Geometry check sheet. Reference: the model listing, model coordinates, mm. A direction names the side the tool comes from. Round coordinates to 2 decimals unless told otherwise and drop trailing zeros. Write each loop counter-clockwise with the first axis right and the second up, starting at its lowest first coordinate (ties: lowest second). Pieces come first, ordered by that corner, then holes. Notation, with made-up numbers: M -24,-39.75 L 9,-39.75 A21 cw 9,-3.75 Z; hole C -5,0.5 d9. An arc over 180 degrees is marked long. One line per item, written item: value. Start each with the question number.
1. Section check D-D (y = -8.5). Record the boundary of the cut face in (x, z).
2. Scan lines: probe 1 along Z at (x, y) = (68.5, -9.25); probe 2 along Z at (x, y) = (0, -7); probe 3 along Z at (x, y) = (46.5, -4). Record each from-to range of solid material in increasing order. Write a range as [from, to].
3. Section check B-B (y = -2.5). Record the boundary of the cut face in (x, z).
4. Section check C-C (z = 0). Record the boundary of the cut face in (x, y).
5. Section check A-A (x = 0). Record the boundary of the cut face in (y, z), and give its area (3 significant figures).
6. Access from +Z, -Z, +X, -X, +Y, -Y to the whole of each face (thin tool, end or side, straight path). Record for faces 1 (the cylindrical face through (54.558, -5.577, -3.722)), 2 (the flat face through (5.766, -2, 0)), 3 (the flat face through (65, -6, -2)).
7. Depth check by flat-ended pin: P1, Ø2, axis at x = 32.5, y = -3.5, coming from the +Z side; P2, Ø5.5, axis at x = 67.5, y = -6.5, coming from the +Z side; P3, Ø5.5, axis at x = 29, y = -7, coming from the -Z side. Enter the tip coordinate at first touch or a pass-through.
8. Release check for a two-part mould opening along Z. For faces 4 (the flat face through (30, -7, 3)), 5 (the flat face through (34, -11, 0)), 6 (the flat face through (65, -6, -5)), 7 (the cylindrical face through (-0.867, -5.423, -3.905)) record: pulls with the +Z half, pulls with the -Z half, needs draft (parallel to the pull), parting line crosses it, or undercut.
from build123d import *

# Parameters (mm, degrees)
F0_R      = 6.5
F0_R_2    = 4
F1_DEPTH  = 15
F3_DEPTH  = 15
F4_W      = 15
F4_H      = 4
F5_DEPTH  = 15
F7_DEPTH  = 15
F8_DEPTH  = 4
F10_DEPTH = 2
F12_DEPTH = 25


with BuildPart() as f1:
    # F0 (on Front) → F1 (new body)
    with BuildSketch(Plane.XZ):
        Circle(F0_R)
        Circle(F0_R_2, mode=Mode.SUBTRACT)
    extrude(amount=F1_DEPTH)

    # F2 (on face) → F3 (join)
    with BuildSketch(Plane.XZ.offset(15)):
        with BuildLine():
            Line((55, 3), (5.7662812973, 3))
            ThreePointArc((5.7662812973, 3), (6.3139064149, 1.5442104078), (6.5, 0))
            ThreePointArc((6.5, 0), (6.3139064149, -1.5442104078), (5.7662812973, -3))
            Line((5.7662812973, -3), (55, -3))
            Line((55, -3), (55, 3))
        make_face()
    extrude(amount=-F3_DEPTH)

    # F4 (on face) → F5 (join)
    with BuildSketch(Plane.XZ.offset(15)):
        Polygon((55, 3), (55, 0), (55, -2), (55, -3), (55, -5), (76, -5), (76, 5), (55, 5), align=None)
        with Locations((65.5, 0)):
            Rectangle(F4_W, F4_H, mode=Mode.SUBTRACT)
    extrude(amount=-F5_DEPTH)

    # F6 (on face) → F7 (join)
    with BuildSketch(Plane.XZ.offset(15)):
        with BuildLine():
            Line((53.3110045666, 3), (52.6317283511, 3))
            ThreePointArc((52.6317283511, 3), (52.9713664589, 2.9713664589), (53.3110045666, 3))
        make_face()
        with BuildLine():
            ThreePointArc((55, 5), (54.5212624717, 3.691116356), (53.3110045666, 3))
            Line((53.3110045666, 3), (55, 3))
            Line((55, 3), (55, 5))
        make_face()
        with BuildLine():
            Line((52.4075180292, -3), (53.4570770231, -3))
            ThreePointArc((53.4570770231, -3), (52.9322975261, -2.9322975261), (52.4075180292, -3))
        make_face()
        with BuildLine():
            ThreePointArc((53.4570770231, -3), (54.569441592, -3.7370064022), (55, -5))
            Line((55, -5), (55, -3))
            Line((55, -3), (53.4570770231, -3))
        make_face()
    extrude(amount=-F7_DEPTH)

    # F8 (cut): a face of the model
    f8_faces = [f1.faces().sort_by_distance(p)[0] for p in [
        (35.8408790092, -15, 0.0001913982),
    ]]
    extrude(f8_faces, amount=-F8_DEPTH, mode=Mode.SUBTRACT)

    # F9 (on face) → F10 (cut)
    with BuildSketch(Plane.XY.offset(5)):
        with BuildLine():
            Line((76, 0), (60.7132725418, 0))
            ThreePointArc((60.7132725418, 0), (67.787035574, -4.3331510207), (76, -5.5))
            Line((76, -5.5), (76, 0))
        make_face()
    extrude(amount=-F10_DEPTH, mode=Mode.SUBTRACT)

    # F11 (on face) → F12 (cut)
    with BuildSketch(Plane.XY.offset(3)):
        Polygon((5.7662812973, 0), (5.7662812973, -3.4528882243), (53.3110045666, 0), align=None)
    extrude(amount=-F12_DEPTH, mode=Mode.SUBTRACT)


solid = f1.part
Result sheet:
1. outline: M 5.77,-3 L 53.46,-3 A2.07 cw 55,-5 L 76,-5 L 76,5 L 55,5 A2.03 cw 53.31,3 L 5.77,3 A6.5 ccw long Z; hole C 0,0 d8; hole M 58,-2 L 73,-2 L 73,2 L 58,2 Z
2. probe 1: z = [-5, -2], [2, 5]
2. probe 2: z = [-6.5, -4], [4, 6.5]
2. probe 3: z = [-3, 3]
3. outline: M 5.77,-3 L 5.77,3 A6.5 ccw long Z; M 18.89,-3 L 53.46,-3 A2.07 cw 55,-5 L 76,-5 L 76,3 L 63.98,3 L 63.98,5 L 55,5 A2.03 cw 53.31,3 L 18.89,3 Z; hole C 0,0 d8; hole M 58,-2 L 73,-2 L 73,2 L 58,2 Z
4. outline: M -6.5,-11 L -4,-11 L -4,0 L -6.5,0 Z; M 4,-11 L 58,-11 L 58,0 L 53.31,0 L 5.77,-3.45 L 5.77,0 L 4,0 Z; M 73,-11 L 76,-11 L 76,0 L 73,0 Z
5. outline: M -11,-6.5 L 0,-6.5 L 0,-4 L -11,-4 Z; M -11,4 L 0,4 L 0,6.5 L -11,6.5 Z
5. area: 55.0 mm2
6. face 1: -Z, +Y, -Y
6. face 2: +Z, -Z, +Y
6. face 3: +Y, -Y
7. P1: stops at z = 3
7. P2: stops at z = 5
7. P3: stops at z = -3
8. face 4: pulls with the +Z half
8. face 5: needs draft
8. face 6: pulls with the -Z half
8. face 7: undercut
